The model under review builds one solid part; all positions refer to its coordinate system, in mm. A direction names the side the tool comes from. Give positions to 0.01 mm unless a question says otherwise; leave off trailing zeros. Write each loop counter-clockwise with the first axis right and the second up, starting at its lowest first coordinate (ties: lowest second). Pieces come first, ordered by that corner, then holes. Notation, with made-up numbers: (22, -39) - (68, -39) arc R29 cw to (68, -2) - close; hole circle Ø4 at (-19, 81). An arc over 180 degrees is marked (long way). Write item = value, one per line.
Autodesk Inventor part; units mm, degrees
ref_plane "Work Plane1" through (0, 112.776, 0) normal (0, 1, 0) x (-1, 0, 0)
ref_plane "YZ Plane" through (0, 0, 0) normal (1, 0, 0) x (0, 1, 0)
ref_plane "XY Plane" through (0, 0, 0) normal (0, 0, 1) x (1, 0, 0)
sketch "Sketch1" plane through (0, 0, 0) normal (0, 1, 0) x (-1, 0, 0)
  line L0 (-12.7, -12.7) -> (12.7, -12.7)
  line L1 (12.7, -12.7) -> (12.7, 12.7)
  line L2 (12.7, 12.7) -> (-12.7, 12.7)
  line L3 (-12.7, 12.7) -> (-12.7, -12.7)
  line L4 (-12.7, -12.7) -> (12.7, 12.7) construction
  line L5 (12.7, -12.7) -> (-12.7, 12.7) construction
  line L6 (9.525, 9.525) -> (9.525, -9.525)
  line L7 (9.525, -9.525) -> (-9.525, -9.525)
  line L8 (-9.525, -9.525) -> (-9.525, 9.525)
  line L9 (-9.525, 9.525) -> (9.525, 9.525)
  point P0 (0, 0)
  dimension "d0" = 25.4
  dimension "d1" = 25.4
  dimension "d2" = 3.175
ref_plane "Work Plane1" through (0, 112.776, 0) normal (0, 1, 0) x (-1, 0, 0)
sketch "Sketch2" plane through (0, 112.776, 0) normal (0, 1, 0) x (-1, 0, 0)
  line L0 (38.1, -12.7) -> (12.7, -12.7)
  line L1 (12.7, -12.7) -> (12.7, 12.7)
  line L2 (12.7, 12.7) -> (38.1, 12.7)
  line L3 (38.1, 12.7) -> (38.1, -12.7)
  line L4 (38.1, -12.7) -> (12.7, 12.7) construction
  line L5 (12.7, -12.7) -> (38.1, 12.7) construction
  line L6 (34.925, 9.525) -> (15.875, 9.525)
  line L7 (15.875, 9.525) -> (15.875, -9.525)
  line L8 (15.875, -9.525) -> (34.925, -9.525)
  line L9 (34.925, -9.525) -> (34.925, 9.525)
  point P0 (0, 0)
  point P1 (25.4, 0)
  point P2 (38.1, 0)
  dimension "d6" = 25.4
  dimension "d7" = 25.4
  dimension "d8" = 3.175
sketch "Sketch3" plane through (0, 0, 0) normal (0, 0, 1) x (1, 0, 0)
  line L0 (-12.7, 112.776) -> (-38.1, 112.776) construction
  line L1 (-25.4, 112.776) -> (0, 0)
sweep "Sweep1" add profiles "Sketch1" path "Sketch3"
properties part number "STRU_006_BilletPole_4.44in"
1. Take a section at A-A on z = 5.25. Give the boundary of the cut face in (x, y) (3 decimals), and give its area (3 significant figures).
Findings below:
outline = (-38.1, 112.776) - (-12.7, 0) - (-9.525, 0) - (-34.925, 112.776) - close; (-15.875, 112.776) - (9.525, 0) - (12.7, 0) - (-12.7, 112.776) - close
area = 716 mm²
2. Insertion check: P1, Ø3, axis at x = -28, y = 54, coming from the +Z side; P2, Ø1.5, axis at y = 22.5, z = 7.5, coming from the +X side; P3, Ø12, axis at y = 81, z = 5, coming from the +X side; P4, Ø3, axis at y = 51, z = -8, coming from the +X side. Each pin has a flat end and moves straight along its axis. Give the tip position at first contact, or say it passes through.
Findings below:
P1 = through
P2 = 7.8
P3 = -4.19
P4 = 1.55
3. For line 1 (Z direction, x = -8, y = 45.5) (3 decimals); line 2 (X direction, y = 27.5, z = -2.5); line 3 (X direction, y = 7, z = 6), list the stretches that pass through material, from the lowest coordinate up. Write a range as from..to.
Findings below:
line_1 = -12.7..-9.525, 9.525..12.7
line_2 = -18.89..-15.72, 3.33..6.51
line_3 = -14.28..-11.1, 7.95..11.12
4. Take a section at D-D on x = -7. Give the boundary of the cut face in (y, z) (3 decimals), and give its area (3 significant figures).
Findings below:
outline = (0, -12.7) - (87.468, -12.7) - (87.468, 12.7) - (0, 12.7) - (0, 9.525) - (73.371, 9.525) - (73.371, -9.525) - (0, -9.525) - close
area = 824 mm²
5. Take a section at B-B on y = 101.5. Give the boundary of the cut face in (x, z) (3 decimals).
Findings below:
outline = (-35.56, -12.7) - (-10.16, -12.7) - (-10.16, 12.7) - (-35.56, 12.7) - close; hole (-32.385, -9.525) - (-13.335, -9.525) - (-13.335, 9.525) - (-32.385, 9.525) - close
6. Draft analysis for pull direction Z (two halves, no side actions). For faces 3 (the flat face through (-25.222, 55.599, -0.178)), 4 (the flat face through (-22.047, 55.599, 0.133)), 5 (the flat face through (-12, 56, -12.7)), state which applies: +Z half, -Z half, draft (parallel to the pull), parting line (faces both ways), or undercut.
Findings below:
face_3 = draft
face_4 = undercut
face_5 = -Z half
7. Take a section at C-C on x = 6. Give the boundary of the cut face in (y, z) (3 decimals), and give its area (3 significant figures).
Findings below:
outline = (0, -12.7) - (29.748, -12.7) - (29.748, 12.7) - (0, 12.7) - (0, 9.525) - (15.651, 9.525) - (15.651, -9.525) - (0, -9.525) - close
area = 457 mm²
8. Machinability: for faces 1 (the flat face through (-2.997, 55.599, -0.133)), 2 (the flat face through (0, 0, 11)), which of the approach directions +Z, -Z, +X, -X, +Y, -Y give a long, thin tool a straight path to every point of the face, cutting with its end or side? Answer none if there is none.
Findings below:
face_1 = none
face_2 = +Z, -Z, +X, -X, -Y
